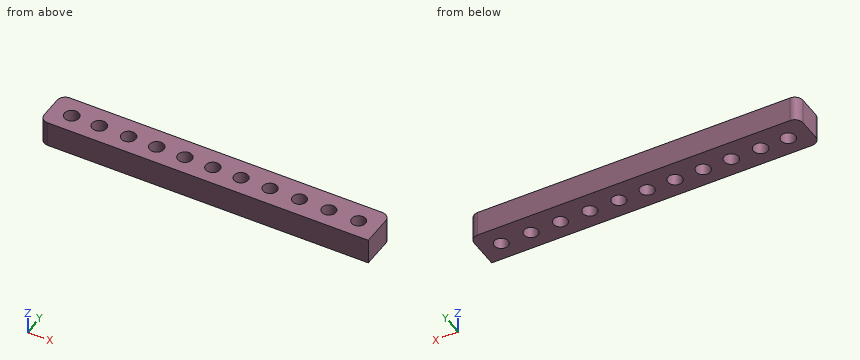
from build123d import *

# Parameters (mm, degrees)
F0_R     = 1.135
F0_R_2   = 1.13
F0_R_3   = 1.125
F0_R_4   = 1.12
F0_R_5   = 1.115
F0_R_6   = 1.11
F0_R_7   = 1.105
F0_R_8   = 1.1
F0_R_9   = 1.095
F0_R_10  = 1.09
F0_R_11  = 1.085
F1_DEPTH = 4


with BuildPart() as f1:
    # F0 (on Top) → F1 (new body)
    with BuildSketch(Plane.XY):
        with BuildLine():
            Line((24.731134, 3.134596), (-24.169983, 3.134596))
            ThreePointArc((-24.169983, 3.134596), (-25.068009, 2.762621), (-25.439983, 1.864596))
            Line((-25.439983, 1.864596), (-25.439983, -1.661713))
            ThreePointArc((-25.439983, -1.661713), (-25.068009, -2.559739), (-24.169983, -2.931713))
            Line((-24.169983, -2.931713), (26.001134, -2.931713))
            Line((26.001134, -2.931713), (26.001134, 1.864596))
            ThreePointArc((26.001134, 1.864596), (25.62916, 2.762621), (24.731134, 3.134596))
        make_face()
        with Locations((-22.08424, 0)):
            Circle(F0_R, mode=Mode.SUBTRACT)
        with Locations((-17.760683, 0)):
            Circle(F0_R_2, mode=Mode.SUBTRACT)
        with Locations((-13.18608, 0)):
            Circle(F0_R_3, mode=Mode.SUBTRACT)
        with Locations((-8.778842, 0)):
            Circle(F0_R_4, mode=Mode.SUBTRACT)
        with Locations((-4.371603, 0)):
            Circle(F0_R_5, mode=Mode.SUBTRACT)
        Circle(F0_R_6, mode=Mode.SUBTRACT)
        with Locations((4.41498, 0)):
            Circle(F0_R_7, mode=Mode.SUBTRACT)
        with Locations((8.961688, 0)):
            Circle(F0_R_8, mode=Mode.SUBTRACT)
        with Locations((13.564184, 0)):
            Circle(F0_R_9, mode=Mode.SUBTRACT)
        with Locations((18.16668, 0)):
            Circle(F0_R_10, mode=Mode.SUBTRACT)
        with Locations((22.824964, 0)):
            Circle(F0_R_11, mode=Mode.SUBTRACT)
    extrude(amount=F1_DEPTH)


solid = f1.part
Verification items for the finished model (mm, model axes). Give positions to 0.01 mm unless a question says otherwise; leave off trailing zeros. Write each loop counter-clockwise with the first axis right and the second up, starting at its lowest first coordinate (ties: lowest second). Pieces come first, ordered by that corner, then holes.
(1) Cross-section at C-C (x = -8.5). Enter the section's corners in (y, z), plus the area to 3 significant figures.
(2) Cross-section at B-B (z = 3.2). State how many separate pieces and enclosed holes the cut face has, plus the area to 3 significant figures.
(3) Cross-section at A-A (x = 0). Enter the section's corners in (y, z), plus the area to 3 significant figures.
(4) Material ranges on line 1 (Y direction, x = -4.5, z = 2.85); line 2 (Y direction, x = 8.5, z = 3.55); line 3 (X direction, y = 2.5, z = 0.65), recorded low to high.
Worked out:
1. outline: (-2.93, 0) - (-1.08, 0) - (-1.08, 4) - (-2.93, 4) - close; (1.08, 0) - (3.13, 0) - (3.13, 4) - (1.08, 4) - close
1. area: 15.6 mm2
2. separate pieces: 1
2. enclosed holes: 11
2. area: 268 mm2
3. outline: (-2.93, 0) - (-1.11, 0) - (-1.11, 4) - (-2.93, 4) - close; (1.11, 0) - (3.13, 0) - (3.13, 4) - (1.11, 4) - close
3. area: 15.4 mm2
4. line 1: y = -2.93 to -1.11, 1.11 to 3.13
4. line 2: y = -2.93 to -1, 1 to 3.13
4. line 3: x = -25.27 to 25.83
